```python
from build123d import *

# Parameters (mm, degrees)
F1_W     = 162.00855
F1_H     = 101.837539
F2_DEPTH = 5
F3_DEPTH = 5.001


with BuildPart() as f2:
    # F1 (on Top) → F2 (new body)
    with BuildSketch(Plane.XY):
        with Locations((45.444982, 10.055467)):
            Rectangle(F1_W, F1_H)
    extrude(amount=F2_DEPTH)

    # F0 (on Top) → F3 (cut, through all)
    with BuildSketch(Plane.XY):
        Polygon((-9.63525, -16.688743), (9.63525, -16.688743), (19.2705, 0), (9.63525, 16.688743), (-9.63525, 16.688743), (-19.2705, 0), align=None)
        Polygon((42.870847, -2.5), (23.600627, -2.5), (13.965517, -19.1885), (23.600627, -35.877), (42.870847, -35.877), (52.505957, -19.1885), align=None)
        Polygon((14.305305, 19.385), (23.940555, 2.696257), (43.211055, 2.696257), (52.846305, 19.385), (43.211055, 36.073743), (23.940555, 36.073743), align=None)
        Polygon((57.176432, -16.492), (76.446652, -16.492), (86.081762, 0.1965), (76.446652, 16.885), (57.176432, 16.885), (47.541322, 0.1965), align=None)
        Polygon((47.88111, 38.77), (57.51636, 22.081257), (76.78686, 22.081257), (86.42211, 38.77), (76.78686, 55.458743), (57.51636, 55.458743), align=None)
        Polygon((90.752237, 2.893), (110.022457, 2.893), (119.657567, 19.5815), (110.022457, 36.27), (90.752237, 36.27), (81.117127, 19.5815), align=None)
    extrude(amount=F3_DEPTH, mode=Mode.SUBTRACT)


solid = f2.part
```
Geometry: final body of the model. Coordinates: model frame, mm. A direction names the side the tool comes from. Coordinates: 2 decimals unless noted, no trailing zeros. Order: outer loops, then holes, each group sorted by start corner. A loop starts at its lowest first (then second) coordinate and runs counter-clockwise, first axis right, second up. Notation, with made-up numbers: (-5.5, -32.5) - (0.5, -32.5) arc R14 ccw to (0.5, -7.5) - close; hole circle Ø9 at (45, 43). An arc over 180 degrees is marked (long way). Write each question's results on one line, items separated by ' | '.
1) Section C-C, the plane x = 16. Return loops of the section in (y, z).
Results list:
outline: (-40.86, 0) - (-22.71, 0) - (-22.71, 5) - (-40.86, 5) - close; (-15.66, 0) - (-5.66, 0) - (-5.66, 5) - (-15.66, 5) - close; (5.66, 0) - (16.45, 0) - (16.45, 5) - (5.66, 5) - close; (22.32, 0) - (60.97, 0) - (60.97, 5) - (22.32, 5) - close
2) Line query: line 1 (Y direction, x = 72, z = 3.25) (3 decimals); line 2 (Y direction, x = 31, z = 2.95); line 3 (Y direction, x = 8, z = 2.1). Output: solid intervals per line, ascending. Write a range as from..to.
Results list:
line 1: -40.863..-16.492, 16.885..22.081, 55.459..60.974 | line 2: -40.86..-35.88, -2.5..2.7, 36.07..60.97 | line 3: -40.86..-16.69, 16.69..60.97
3) Section B-B, the plane y = -6. Return loops of the section in (x, z).
Results list:
outline: (-35.56, 0) - (-15.81, 0) - (-15.81, 5) - (-35.56, 5) - close; (15.81, 0) - (21.58, 0) - (21.58, 5) - (15.81, 5) - close; (44.89, 0) - (51.12, 0) - (51.12, 5) - (44.89, 5) - close; (82.5, 0) - (126.45, 0) - (126.45, 5) - (82.5, 5) - close
4) Pull-direction query (Y, two-part tool) for faces 3 (the flat face through (126.449, 9, 2)), 4 (the flat face through (67, 16.885, 2)), 5 (the flat face through (44, -40.863, 2)), 6 (the flat face through (44, 60.974, 2)); classes: pulls with the +Y half, pulls with the -Y half, needs draft (parallel to the pull), parting line crosses it, or undercut.
Results list:
face 3: needs draft | face 4: undercut | face 5: pulls with the -Y half | face 6: pulls with the +Y half
5) Section D-D, the plane y = 10. Return loops of the section in (x, z), plus the area to 3 significant figures.
Results list:
outline: (-35.56, 0) - (-13.5, 0) - (-13.5, 5) - (-35.56, 5) - close; (13.5, 0) - (19.72, 0) - (19.72, 5) - (13.5, 5) - close; (47.43, 0) - (53.2, 0) - (53.2, 5) - (47.43, 5) - close; (80.42, 0) - (86.65, 0) - (86.65, 5) - (80.42, 5) - close; (114.13, 0) - (126.45, 0) - (126.45, 5) - (114.13, 5) - close | area: 263 mm^2
6) Section A-A, the plane x = 108. Return loops of the section in (y, z), plus the area to 3 significant figures.
Results list:
outline: (-40.86, 0) - (2.89, 0) - (2.89, 5) - (-40.86, 5) - close; (36.27, 0) - (60.97, 0) - (60.97, 5) - (36.27, 5) - close | area: 342 mm^2
7) Set-up query: faces 1 (the flat face through (44, -1, 5)), 2 (the flat face through (81.54, 30.31, 2.46)). Return all of +Z, -Z, +X, -X, +Y, -Y with unobstructed straight access to the full face (end or side cutting, diameter ignored); none if empty.
Results list:
face 1: +Z, +X, -X, +Y, -Y | face 2: +Z, -Z
